The model under review builds one solid part; all positions refer to its coordinate system, in mm. A direction names the side the tool comes from. Give positions to 0.01 mm unless a question says otherwise; leave off trailing zeros. Loops run counter-clockwise (first coordinate to the right, second up) from the corner with the lowest first, then second, coordinate; pieces in that order, holes last. Notation, with made-up numbers: M 63,76 L 120,76 A22 cw 120,96 Z; hole C 47,60 d2. An arc over 180 degrees is marked long. Return JSON: item names as keys, results as strings.
```python
from build123d import *

# Parameters (mm, degrees)
F1_DEPTH = 60
F2_R     = 2.6
F3_DEPTH = 25
F4_R     = 2
F5_W     = 45
F5_H     = 8
F6_DEPTH = 8
F7_R     = 2.6
F8_DEPTH = 50
F9_R     = 1


with BuildPart() as f1:
    # F0 (on Front) → F1 (new body)
    with BuildSketch(Plane.XZ):
        with BuildLine():
            ThreePointArc((12.5, 0), (0, -12.5), (-12.5, 0))
            Line((-12.5, 0), (-22.5, 0))
            Line((-22.5, 0), (-22.5, -16))
            Line((-22.5, -16), (22.5, -16))
            Line((22.5, -16), (22.5, 0))
            Line((22.5, 0), (12.5, 0))
        make_face()
    extrude(amount=F1_DEPTH)

    # F2 (on face) → F3 (cut)
    with BuildSketch(Plane.XY):
        with Locations((-17.5, -50)):
            Circle(F2_R)
        with Locations((-17.5, -10)):
            Circle(F2_R)
        with Locations((17.5, -50)):
            Circle(F2_R)
        with Locations((17.5, -10)):
            Circle(F2_R)
    extrude(amount=-F3_DEPTH, mode=Mode.SUBTRACT)

    # F4
    f4_edges = [f1.edges().sort_by_distance(p)[0] for p in [
        (0, -60, -12.5),
        (0, 0, -12.5),
    ]]
    fillet(f4_edges, radius=F4_R)

    # F5 (on face) → F6 (join)
    with BuildSketch(Plane(origin=(0, 0, -16), x_dir=(1, 0, 0), z_dir=(0, 0, -1))):
        with Locations((0, 21.5)):
            Rectangle(F5_W, F5_H)
        with Locations((0, 38.5)):
            Rectangle(F5_W, F5_H)
    extrude(amount=F6_DEPTH)

    # F7 (on face) → F8 (cut)
    with BuildSketch(Plane(origin=(-22.5, 0, 0), x_dir=(0, -1, 0), z_dir=(-1, 0, 0))):
        with Locations((38.5, -20)):
            Circle(F7_R)
        with Locations((21.5, -20)):
            Circle(F7_R)
    extrude(amount=-F8_DEPTH, mode=Mode.SUBTRACT)

    # F9
    f9_edges = [f1.edges().sort_by_distance(p)[0] for p in [
        (0, -17.5, -24),
        (0, -17.5, -16),
        (0, -25.5, -24),
        (0, -25.5, -16),
        (0, -34.5, -16),
        (0, -34.5, -24),
        (0, -42.5, -24),
        (0, -42.5, -16),
    ]]
    fillet(f9_edges, radius=F9_R)


solid = f1.part
```
1) Consider section D-D on x = 0. Write out the cut boundary in (y, z).
From the geometry:
{"outline": "M -60,-16 L -43.5,-16 A1 cw -42.5,-17 L -42.5,-23 A1 ccw -41.5,-24 L -35.5,-24 A1 ccw -34.5,-23 L -34.5,-17 A1 cw -33.5,-16 L -26.5,-16 A1 cw -25.5,-17 L -25.5,-23 A1 ccw -24.5,-24 L -18.5,-24 A1 ccw -17.5,-23 L -17.5,-17 A1 cw -16.5,-16 L 0,-16 L 0,-14.5 A2 ccw -2,-12.5 L -58,-12.5 A2 ccw -60,-14.5 Z; hole C -38.5,-20 d5.2; hole C -21.5,-20 d5.2"}
2) Consider section A-A on x = 17.5. Count the separate pieces of the cut face and the enclosed holes in it, then the cut area to 3 significant figures.
From the geometry:
{"separate pieces": "3", "enclosed holes": "2", "area": "879 mm²"}
3) Consider section C-C on y = -21.5. Write out the cut boundary in (x, z).
From the geometry:
{"outline": "M -22.5,-24 L 22.5,-24 L 22.5,-22.6 L -22.5,-22.6 Z; M -22.5,-17.4 L 22.5,-17.4 L 22.5,0 L 12.5,0 A12.5 cw -12.5,0 L -22.5,0 Z"}
4) Consider section B-B on y = -50. Write out the cut boundary in (x, z).
From the geometry:
{"outline": "M -22.5,-16 L -20.1,-16 L -20.1,0 L -22.5,0 Z; M -14.9,-16 L 14.9,-16 L 14.9,0 L 12.5,0 A12.5 cw -12.5,0 L -14.9,0 Z; M 20.1,-16 L 22.5,-16 L 22.5,0 L 20.1,0 Z"}
5) Tool access review of faces 1 (the face through (18, -30, 0)), 2 (the face through (0, -34.5, -20)), 3 (the face through (0, -52, -16)), 4 (the face through (0, -8, -16)): name each direction out of +Z, -Z, +X, -X, +Y, -Y from which nothing blocks a thin tool from reaching the whole face with its end or side.
From the geometry:
{"face 1": "+Z, +X, -X, +Y, -Y", "face 2": "-Z, +X, -X", "face 3": "-Z, +X, -X, -Y", "face 4": "-Z, +X, -X, +Y"}
6) The part is to be moulded in two halves that separate along Z. For faces 5 (the face through (0, -25.5, -20)), 6 (the face through (0, -30, -16)), 7 (the face through (-0.32, -22.9, -17.81)), say which applies: released by +Z, released by -Z, zero draft, split by the parting line, or undercut.
From the geometry:
{"face 5": "zero draft", "face 6": "released by -Z", "face 7": "undercut"}
7) Insertion check: pin 1 (1.8 mm diameter, centred on x = 0.5, z = -20.5, fed in from -Y); pin 2 (2 mm diameter, centred on x = 15, y = -48, fed in from -Z); pin 3 (1.5 mm diameter, centred on x = 14.5, z = -13.5, fed in from +Y); pin 4 (4 mm diameter, centred on x = 3.5, y = -13.5, fed in from +Z) (3 decimals). Each pin has a flat end and moves straight along its axis. Give the tip position at first contact, or say it passes through.
From the geometry:
{"pin 1": "y = -42.5", "pin 2": "z = -16", "pin 3": "y = 0", "pin 4": "z = -11.225"}
8) Wall thickness on L1, parallel to Y at x = -17.5, z = -7.75; L2, parallel to Z at x = 17, y = -33; L3, parallel to X at y = -25, z = -2.25: over which ranges is each line inside the solid? List them lowest first. Write a range as from..to.
From the geometry:
{"L1": "-60..-52.6, -47.4..-12.6, -7.4..0", "L2": "-16..0", "L3": "-22.5..-12.3, 12.3..22.5"}
